Input: part model. Units: mm. Frame: model coordinates. A direction names the side the tool comes from. Coordinates: 2 decimals unless noted, no trailing zeros. Order: outer loops, then holes, each group sorted by start corner. A loop starts at its lowest first (then second) coordinate and runs counter-clockwise, first axis right, second up. Notation, with made-up numbers: (-17, 48) - (18, 48) arc R28 cw to (18, 79) - close; hole circle Ø11 at (59.25, -39). An arc over 180 degrees is marked (long way). One line per question, with ' | ' between items.
from build123d import *

# Parameters (mm, degrees)
EXTRUDE_1_DEPTH     = 4
SKETCH_2_R          = 1.6
CUT_EXTRUDE_1_DEPTH = 72.700767081
SKETCH_3_R          = 2
SKETCH_3_R_2        = 1.6
CUT_EXTRUDE_2_DEPTH = 72.700767081
SKETCH_4_W          = 130
SKETCH_4_H          = 2
EXTRUDE_2_DEPTH     = 4
FILLET_1_R          = 7


with BuildPart() as part:
    # 草图1 → 凸台-拉伸1 (new body)
    with BuildSketch(Plane(origin=(0, 0, 0), x_dir=(1, 0, 0), z_dir=(0, 1, 0))):
        Polygon((25, 0), (-25, 0), (-65, 15), (-65, 30), (65, 30), (65, 15), align=None)
    extrude(amount=EXTRUDE_1_DEPTH)

    # 草图2 → 切除-拉伸1 (cut, through all)
    with BuildSketch(Plane(origin=(0, 4, 0), x_dir=(1, 0, 0), z_dir=(0, 1, 0))):
        with Locations(Location((-7.5, 18, 0), (0, 0, 270))):
            Circle(SKETCH_2_R)
        with Locations(Location((7.5, 18, 0), (0, 0, 90))):
            Circle(SKETCH_2_R)
        with Locations(Location((-7.5, 8, 0), (0, 0, 90))):
            Circle(SKETCH_2_R)
        with Locations(Location((7.5, 8, 0), (0, 0, 270))):
            Circle(SKETCH_2_R)
    extrude(amount=-CUT_EXTRUDE_1_DEPTH, mode=Mode.SUBTRACT)

    # 草图3 → 切除-拉伸2 (cut, through all)
    with BuildSketch(Plane(origin=(0, 4, 0), x_dir=(1, 0, 0), z_dir=(0, 1, 0))):
        with Locations(Location((-58, 22, 0), (0, 0, 270))):
            Circle(SKETCH_3_R)
        with Locations(Location((58, 22, 0), (0, 0, 90))):
            Circle(SKETCH_3_R)
        with Locations(Location((-13.5, 5, 0), (0, 0, 270))):
            Circle(SKETCH_3_R_2)
        with Locations(Location((-13.5, 25, 0), (0, 0, 270))):
            Circle(SKETCH_3_R_2)
        with Locations(Location((13.5, 5, 0), (0, 0, 90))):
            Circle(SKETCH_3_R_2)
        with Locations(Location((13.5, 25, 0), (0, 0, 90))):
            Circle(SKETCH_3_R_2)
        with BuildLine():
            Line((-51, 23.236030392), (-51, 15.857143498))
            ThreePointArc((-51, 15.857143498), (-50.793424544, 15.248474875), (-50.259045015, 14.891278248))
            Line((-50.259045015, 14.891278248), (-27.921339757, 8.900306744))
            ThreePointArc((-27.921339757, 8.900306744), (-26.741501421, 9.476121152), (-27.148724711, 10.724219675))
            Line((-27.148724711, 10.724219675), (-49.486429968, 24.094078073))
            ThreePointArc((-49.486429968, 24.094078073), (-50.493168312, 24.105964306), (-51, 23.236030392))
        make_face()
        with BuildLine():
            Line((-38.782523044, 22.349179917), (-25.724953573, 14.533790966))
            ThreePointArc((-25.724953573, 14.533790966), (-24.718215229, 14.521904732), (-24.211383541, 15.391838647))
            Line((-24.211383541, 15.391838647), (-24.211383541, 21.145506102))
            ThreePointArc((-24.211383541, 21.145506102), (-24.451132736, 21.795135776), (-25.055420968, 22.133269067))
            Line((-25.055420968, 22.133269067), (-38.112990439, 24.194990563))
            ThreePointArc((-38.112990439, 24.194990563), (-39.209019504, 23.548218787), (-38.782523044, 22.349179917))
        make_face()
        with BuildLine():
            Line((-10.229137867, 12.546046067), (-17.517122215, 19.57620297))
            ThreePointArc((-17.517122215, 19.57620297), (-18.602368626, 19.776876975), (-19.211383541, 18.856479961))
            Line((-19.211383541, 18.856479961), (-19.211383541, 8.182330884))
            ThreePointArc((-19.211383541, 8.182330884), (-18.737114654, 7.331680075), (-17.764169946, 7.287903693))
            Line((-17.764169946, 7.287903693), (-10.476185598, 10.931895866))
            ThreePointArc((-10.476185598, 10.931895866), (-9.934909706, 11.67503349), (-10.229137867, 12.546046067))
        make_face()
        with BuildLine():
            Line((17.764169946, 7.287903693), (10.476185598, 10.931895866))
            ThreePointArc((10.476185598, 10.931895866), (9.934909706, 11.67503349), (10.229137867, 12.546046067))
            Line((10.229137867, 12.546046067), (17.517122215, 19.57620297))
            ThreePointArc((17.517122215, 19.57620297), (18.602368626, 19.776876975), (19.211383541, 18.856479961))
            Line((19.211383541, 18.856479961), (19.211383541, 8.182330884))
            ThreePointArc((19.211383541, 8.182330884), (18.737114654, 7.331680075), (17.764169946, 7.287903693))
        make_face()
        with BuildLine():
            Line((25.055420968, 22.133269067), (38.112990439, 24.194990563))
            ThreePointArc((38.112990439, 24.194990563), (39.209019504, 23.548218787), (38.782523044, 22.349179917))
            Line((38.782523044, 22.349179917), (25.724953573, 14.533790966))
            ThreePointArc((25.724953573, 14.533790966), (24.718215229, 14.521904732), (24.211383541, 15.391838647))
            Line((24.211383541, 15.391838647), (24.211383541, 21.145506102))
            ThreePointArc((24.211383541, 21.145506102), (24.451132736, 21.795135776), (25.055420968, 22.133269067))
        make_face()
        with BuildLine():
            Line((27.148724711, 10.724219675), (49.486429968, 24.094078073))
            ThreePointArc((49.486429968, 24.094078073), (50.493168312, 24.105964306), (51, 23.236030392))
            Line((51, 23.236030392), (51, 15.857143498))
            ThreePointArc((51, 15.857143498), (50.793424544, 15.248474875), (50.259045015, 14.891278248))
            Line((50.259045015, 14.891278248), (27.921339757, 8.900306744))
            ThreePointArc((27.921339757, 8.900306744), (26.741501421, 9.476121152), (27.148724711, 10.724219675))
        make_face()
    extrude(amount=-CUT_EXTRUDE_2_DEPTH, mode=Mode.SUBTRACT)

    # 草图4 → 凸台-拉伸2 (add)
    with BuildSketch(Plane(origin=(0, 4, 0), x_dir=(1, 0, 0), z_dir=(0, 1, 0))):
        with Locations((0, 31)):
            Rectangle(SKETCH_4_W, SKETCH_4_H)
    extrude(amount=-EXTRUDE_2_DEPTH)

    # 圆角1
    fillet_1_edges = [part.edges().sort_by_distance(p)[0] for p in [
        (-65, 2, -15),
        (65, 2, -15),
        (25, 2, 0),
        (-25, 2, 0),
        (-65, 2, -32),
        (65, 2, -32),
    ]]
    fillet(fillet_1_edges, radius=FILLET_1_R)


solid = part.part
Item 1: Section D-D on z = -29.5. Return the cut outline in (x, y).
Data:
outline: (-63.36, 0) - (63.36, 0) - (63.36, 4) - (-63.36, 4) - close
Item 2: Draft query along X for faces 1 (the face through (-63, 2, -29.9)), 2 (the face through (51, 2, -20)), 3 (the face through (24.997, 2.028, -0.115)). Return one class per face: released by +X, released by -X, zero draft, split by the parting line, or undercut.
Data:
face 1: released by -X | face 2: undercut | face 3: released by +X
Item 3: Section B-B on z = -5. Return the cut outline in (x, y).
Data:
outline: (-38.33, 0) - (-15.1, 0) - (-15.1, 4) - (-38.33, 4) - close; (-11.9, 0) - (11.9, 0) - (11.9, 4) - (-11.9, 4) - close; (15.1, 0) - (38.33, 0) - (38.33, 4) - (15.1, 4) - close
Item 4: Section C-C on y = 3.1. Count the separate pieces of the cut face and the enclosed holes in it, and give its area (3 significant figures).
Data:
separate pieces: 1 | enclosed holes: 16 | area: 2,860 mm^2
Item 5: Ray query, line 1 (X direction, y = 1.4, z = -26); line 2 (Z direction, x = 32, y = 0.75) (3 decimals); line 3 (X direction, y = 2.5, z = -25.5). Return the intervals inside material, ascending.
Data:
line 1: -64.93 to -14.75, -12.25 to 12.25, 14.75 to 64.93 | line 2: -32 to -23.23, -18.29 to -13.628, -9.994 to -2.625 | line 3: -64.98 to -15.02, -11.98 to 11.98, 15.02 to 64.98
Item 6: Access query for faces 4 (the face through (31.49, 2.03, -23.15)), 5 (the face through (-1, 0, -20)). Directions: +Z, -Z, +X, -X, +Y, -Y. A direction counts if a zero-diameter tool reaches every point of the face in a straight line with its end or side. Return the directions, or none.
Data:
face 4: +Y, -Y | face 5: +Z, -Z, +X, -X, -Y
Item 7: Contact query for flat-ended pins moving along their axis: P1, Ø5, axis at x = 7.5, z = -8, coming from the -Y side; P2, Ø2, axis at y = 0.5, z = -14.5, coming from the +X side. Output: stop coordinate, or through.
Data:
P1: y = 0 | P2: x = 63.48
Item 8: Section A-A on x = 7.5. Return the cut outline in (y, z), and give its area (3 significant figures).
Data:
outline: (0, -32) - (4, -32) - (4, -19.6) - (0, -19.6) - close; (0, -16.4) - (4, -16.4) - (4, -9.6) - (0, -9.6) - close; (0, -6.4) - (4, -6.4) - (4, 0) - (0, 0) - close | area: 102 mm^2
